from build123d import *

# Parameters (mm, degrees)
SKETCH1_R               = 20
BOSS_EXTRUDE1_DEPTH     = 10
SKETCH2_R               = 30
BOSS_EXTRUDE2_DEPTH     = 10
BOSS_EXTRUDE3_START     = 10
SKETCH3_R               = 30
BOSS_EXTRUDE3_DEPTH     = 10
SKETCH9_R               = 30
BOSS_EXTRUDE7_DEPTH     = 30
CUT_EXTRUDE1_DEPTH      = 56
CUT_EXTRUDE1_DEPTH_BACK = 56
SKETCH13_R              = 36.178766014
SKETCH13_R_2            = 30
SKETCH14_W              = 9.580398915
SKETCH14_H              = 10
CUT_REVOLVE6_ANGLE      = 180


with BuildPart() as part:
    # Sketch1 → Boss-Extrude1 (new body)
    with BuildSketch(Plane(origin=(0, 0, 0), x_dir=(1, 0, 0), z_dir=(0, 1, 0))):
        with Locations(Location((0, 0, 0), (0, 0, 270))):
            Circle(SKETCH1_R)
    extrude(amount=BOSS_EXTRUDE1_DEPTH)

    # Sketch2 → Boss-Extrude2 (add)
    with BuildSketch(Plane(origin=(0, 10, 0), x_dir=(1, 0, 0), z_dir=(0, 1, 0))):
        with Locations(Location((0, 0, 0), (0, 0, 270))):
            Circle(SKETCH2_R)
    extrude(amount=BOSS_EXTRUDE2_DEPTH)

    # Sketch3 → Boss-Extrude3 (add)
    with BuildSketch(Plane.XZ.offset(BOSS_EXTRUDE3_START)):
        with Locations(Location((0, 0, 0), (0, 0, 90))):
            Circle(SKETCH3_R)
    extrude(amount=-BOSS_EXTRUDE3_DEPTH)

    # Sketch9 → Boss-Extrude7 (add)
    with BuildSketch(Plane.XY):
        with Locations((0, 5)):
            Circle(SKETCH9_R)
    extrude(amount=-BOSS_EXTRUDE7_DEPTH)

    # Sketch13 → Cut-Extrude1 (cut, two sides: drawn at the far end of the back side and taken through both)
    with BuildSketch(Plane.XY.offset(-CUT_EXTRUDE1_DEPTH_BACK)):
        with Locations((0, 5)):
            Circle(SKETCH13_R)
        with Locations((0, 5)):
            Circle(SKETCH13_R_2, mode=Mode.SUBTRACT)
    extrude(amount=CUT_EXTRUDE1_DEPTH + CUT_EXTRUDE1_DEPTH_BACK, mode=Mode.SUBTRACT)

    # Sketch14 → Cut-Revolve6 (revolve, cut)
    with BuildSketch(Plane.XY):
        with Locations((24.790199458, 5)):
            Rectangle(SKETCH14_W, SKETCH14_H)
    revolve(axis=Axis((0, 0, 0), (0, 1, 0)), revolution_arc=CUT_REVOLVE6_ANGLE, mode=Mode.SUBTRACT)


solid = part.part
The model under review builds one solid part; all positions refer to its coordinate system, in mm. A direction names the side the tool comes from. Give positions to 0.01 mm unless a question says otherwise; leave off trailing zeros. Order: outer loops, then holes, each group sorted by start corner. A loop starts at its lowest first (then second) coordinate and runs counter-clockwise, first axis right, second up. Notation, with made-up numbers: M 48.5,-26 L 74.5,-26 A5 ccw 74.5,-17 Z; hole C 66.25,-20.75 d9. An arc over 180 degrees is marked long. Answer in a Markdown table with one row per item. Add a question column.
1. Add section C-C on z = -25.5. State the section outline as (x, y) points, plus the area to 3 significant figures.
2. For pin 1 Ø10 at (x, z) = (14.5, -1) entering from +Y; pin 2 Ø0.5 at (x, y) = (-30, 5.5) entering from +Z; pin 3 Ø3 at (x, z) = (-3, -17) entering from -Y, all flat-tipped, find the tip position at first contact; note any pin that passes through.
3. Add section D-D on x = -25. State the section outline as (y, z) points.
4. Add section A-A on y = 5. State the section outline as (x, z) points.
5. Add section B-B on x = 0. State the section outline as (y, z) points, plus the area to 3 significant figures.
6. Machinability: for faces 1 (the cylindrical face through (-16, 5, 12)), 2 (the flat face through (0, 5, -30)), which of the approach directions +Z, -Z, +X, -X, +Y, -Y give a long, thin tool a straight path to every point of the face, cutting with its end or side? Answer none if there is none.
7. To check wall thickness, follow line 1 along Y through (x, z) = (-6, 19.5); line 2 along Y through (x, z) = (14.5, 9); line 3 along Z through (x, y) = (23, 23). State the ranges of each line that lie inside material, in increasing order.
8. Mouldability with a two-part tool opening along Z and no side actions: class faces 3 (the cylindrical face through (0.65, 5.07, -29.573)), 4 (the flat face through (0, 20, 11)), 5 (the flat face through (0, -16, 0)) as released by +Z, released by -Z, zero draft, split by the parting line, or undercut.
The answers:
| question | item | result |
|---|---|---|
| 1 | outline | C 0,5 d60; hole M -14.99,0 L 14.99,0 L 14.99,10 L -14.99,10 Z |
| 1 | area | 2,530 mm2 |
| 2 | pin 1 | y = 33.46 |
| 2 | pin 2 | z = 0 |
| 2 | pin 3 | y = -24.96 |
| 3 | outline | M -11.58,-30 L 21.58,-30 L 21.58,0 L 20,0 L 20,16.58 L 10,16.58 L 10,-15.81 L 0,-15.81 L 0,16.58 L -10,16.58 L -10,0 L -11.58,0 Z |
| 4 | outline | M -30,-30 L 30,-30 L 30,0 L 29.58,0 A29.58 cw -29.58,0 L -30,0 Z; C 0,0 d40 |
| 5 | outline | M -25,-30 L 35,-30 L 35,0 L 20,0 L 20,30 L 10,30 L 10,20 L 0,20 L 0,30 L -10,30 L -10,0 L -25,0 Z; hole M 0,-29.58 L 10,-29.58 L 10,-20 L 0,-20 Z |
| 5 | area | 2,500 mm2 |
| 6 | face 1 | none |
| 6 | face 2 | -Z, +X, -X, +Y, -Y |
| 7 | line 1 | -10 to 0, 10 to 20 |
| 7 | line 2 | -10 to 20 |
| 7 | line 3 | -30 to 0 |
| 8 | face 3 | undercut |
| 8 | face 4 | zero draft |
| 8 | face 5 | released by +Z |
